from build123d import *

# Parameters (mm, degrees)
BOSS_EXTRUDE1_DEPTH = 4
SKETCH2_R           = 1.6
CUT_EXTRUDE1_DEPTH  = 5
SKETCH3_W           = 25
SKETCH3_H           = 4
CUT_EXTRUDE2_DEPTH  = 5
BOSS_EXTRUDE2_DEPTH = 25


with BuildPart() as part:
    # Sketch1 → Boss-Extrude1 (new body)
    with BuildSketch(Plane(origin=(0, 0, 0), x_dir=(1, 0, 0), z_dir=(0, 1, 0))):
        with BuildLine():
            Line((0, 5), (55, 5))
            ThreePointArc((55, 5), (60, 0), (55, -5))
            Line((55, -5), (0, -5))
            ThreePointArc((0, -5), (-5, 0), (0, 5))
        make_face()
    extrude(amount=BOSS_EXTRUDE1_DEPTH)

    # Sketch2 → Cut-Extrude1 (cut, through all)
    with BuildSketch(Plane(origin=(0, 4, 0), x_dir=(1, 0, 0), z_dir=(0, 1, 0))):
        Circle(SKETCH2_R)
        with Locations((27.5, 0)):
            Circle(SKETCH2_R)
    extrude(amount=-CUT_EXTRUDE1_DEPTH, mode=Mode.SUBTRACT)

    # Sketch3 → Cut-Extrude2 (cut)
    with BuildSketch(Plane(origin=(0, 0, -5), x_dir=(-1, 0, 0), z_dir=(0, 0, -1))):
        with Locations((-42.5, 2)):
            Rectangle(SKETCH3_W, SKETCH3_H)
    extrude(amount=-CUT_EXTRUDE2_DEPTH, mode=Mode.SUBTRACT)

    # Sketch4 → Boss-Extrude2 (add)
    with BuildSketch(Plane.ZY.offset(-55)):
        Polygon((0, 4), (-5, 0), (0, 0), align=None)
    extrude(amount=BOSS_EXTRUDE2_DEPTH)


solid = part.part
Can you work these out from the model? Positions are in its coordinate system, mm. A direction names the side the tool comes from. Coordinates: 2 decimals unless noted, no trailing zeros. Write each loop counter-clockwise with the first axis right and the second up, starting at its lowest first coordinate (ties: lowest second). Pieces come first, ordered by that corner, then holes. Notation, with made-up numbers: (24, -18) -> (75, -18) arc R30 ccw to (75, 8) -> close; hole circle Ø8 at (18, 37). An arc over 180 degrees is marked (long way). Write item = value, one per line.
(1) Imagine slicing it at A-A (x = 27.5). Please give me the cut outline in (y, z), and give its area (3 significant figures).
Verdict:
outline = (0, -5) -> (4, -5) -> (4, -1.6) -> (0, -1.6) -> close; (0, 1.6) -> (4, 1.6) -> (4, 5) -> (0, 5) -> close
area = 27.2 mm^2
(2) Thinking about a two-plate mould opening in Z: for faces 3 (the face through (28, 0, 2)), 4 (the face through (15, 2, -5)), 5 (the face through (26.32, 2.03, -1.08)), which applies, +Z half, -Z half, draft (parallel to the pull), parting line (faces both ways), or undercut?
Verdict:
face_3 = draft
face_4 = -Z half
face_5 = undercut
(3) Imagine slicing it at B-B (y = 0.8). Please give me the cut outline in (x, z), and give its area (3 significant figures).
Verdict:
outline = (0, -5) -> (30, -5) -> (30, -4) -> (55, -4) -> (55, -5) arc R5 ccw to (55, 5) -> (0, 5) arc R5 ccw to start; hole circle Ø3.2 at (0, 0); hole circle Ø3.2 at (27.5, 0)
area = 587 mm^2
(4) On a 3-axis mill with a long thin cutter (end or side, diameter ignored), from which of +Z, -Z, +X, -X, +Y, -Y can I reach the whole of each face in a straight line? I mean faces 1 (the face through (30, 3, -4)), 2 (the face through (28, 2, 5)). Say none if no direction works.
Verdict:
face_1 = -Z, +Y
face_2 = +Z, +X, -X, +Y, -Y
(5) If I drill on probe 1 along X at (y, z) = (1.8, 0); probe 2 along Z at (x, y) = (0, 2.9); probe 3 along X at (y, z) = (1.9, -3), over which ranges is the centre line in solid material (lowest first)?
Verdict:
probe_1 = -5 to -1.6, 1.6 to 25.9, 29.1 to 60
probe_2 = -5 to -1.6, 1.6 to 5
probe_3 = -4 to 30, 55 to 59
(6) For pin 1 (2 mm diameter, centred on y = 3, z = -1.5, fed in from -X); pin 2 (1.5 mm diameter, centred on x = 45.5, y = 2.5, fed in from -Z), each with a flat end and sliding along its axis, tell me the tip position at first contact or that it passes through.
Verdict:
pin_1 = -4.97
pin_2 = -2.81
(7) Imagine slicing it at C-C (z = 1). Please give me the cut outline in (x, y).
Verdict:
outline = (-4.9, 0) -> (-1.25, 0) -> (-1.25, 4) -> (-4.9, 4) -> close; (1.25, 0) -> (26.25, 0) -> (26.25, 4) -> (1.25, 4) -> close; (28.75, 0) -> (59.9, 0) -> (59.9, 4) -> (28.75, 4) -> close
(8) Imagine slicing it at D-D (z = -4.25). Please give me the cut outline in (x, y), and give its area (3 significant figures).
Verdict:
outline = (-2.63, 0) -> (57.63, 0) -> (57.63, 4) -> (55, 4) -> (55, 0.6) -> (30, 0.6) -> (30, 4) -> (-2.63, 4) -> close
area = 156 mm^2
